```python
from build123d import *

# Parameters (mm, degrees)
SKETCH_1_W          = 10
SKETCH_1_H          = 10
EXTRUDE_1_DEPTH     = 2
EXTRUDE_2_DEPTH     = 3.3
SKETCH_3_R          = 2
CUT_EXTRUDE_1_DEPTH = 3.3
SKETCH_4_R          = 0.75
CUT_EXTRUDE_2_DEPTH = 3.3
SKETCH_5_R          = 1.5
CUT_EXTRUDE_3_DEPTH = 1
CUT_EXTRUDE_4_DEPTH = 9.836854644


with BuildPart() as part:
    # 草图1 → 凸台-拉伸1 (new body)
    with BuildSketch(Plane(origin=(0, 0, 0), x_dir=(1, 0, 0), z_dir=(0, 1, 0))):
        Rectangle(SKETCH_1_W, SKETCH_1_H)
    extrude(amount=EXTRUDE_1_DEPTH)

    # 草图2 → 凸台-拉伸2 (add)
    with BuildSketch(Plane.XZ):
        with BuildLine():
            ThreePointArc((-3.353126844, -0.498638517), (-2.397091988, -2.397091988), (-0.498638517, -3.353126844))
            ThreePointArc((-0.498638517, -3.353126844), (0, -2.89), (0.498638517, -3.353126844))
            ThreePointArc((0.498638517, -3.353126844), (2.397091988, -2.397091988), (3.353126844, -0.498638517))
            ThreePointArc((3.353126844, -0.498638517), (2.89, 0), (3.353126844, 0.498638517))
            ThreePointArc((3.353126844, 0.498638517), (2.397091988, 2.397091988), (0.498638517, 3.353126844))
            ThreePointArc((0.498638517, 3.353126844), (0, 2.89), (-0.498638517, 3.353126844))
            ThreePointArc((-0.498638517, 3.353126844), (-2.397091988, 2.397091988), (-3.353126844, 0.498638517))
            ThreePointArc((-3.353126844, 0.498638517), (-2.89, 0), (-3.353126844, -0.498638517))
        make_face()
    extrude(amount=EXTRUDE_2_DEPTH)

    # 草图3 → 切除-拉伸1 (cut)
    with BuildSketch(Plane.XZ.offset(3.3)):
        with Locations(Location((0, 0, 0), (0, 0, 270))):
            Circle(SKETCH_3_R)
    extrude(amount=-CUT_EXTRUDE_1_DEPTH, mode=Mode.SUBTRACT)

    # 草图4 → 切除-拉伸2 (cut)
    with BuildSketch(Plane.XZ):
        with Locations(Location((0, 0, 0), (0, 0, 270))):
            Circle(SKETCH_4_R)
    extrude(amount=-CUT_EXTRUDE_2_DEPTH, mode=Mode.SUBTRACT)

    # 草图5 → 切除-拉伸3 (cut)
    with BuildSketch(Plane(origin=(0, 2, 0), x_dir=(1, 0, 0), z_dir=(0, 1, 0))):
        with Locations(Location((0, 0, 0), (0, 0, 270))):
            Circle(SKETCH_5_R)
    extrude(amount=-CUT_EXTRUDE_3_DEPTH, mode=Mode.SUBTRACT)

    # 草图6 → 切除-拉伸4 (cut, through all)
    with BuildSketch(Plane(origin=(0, 2, 0), x_dir=(1, 0, 0), z_dir=(0, 1, 0))):
        with BuildLine():
            Line((-0.5, 5), (0.5, 5))
            ThreePointArc((0.5, 5), (0, 4.5), (-0.5, 5))
        make_face()
    extrude(amount=-CUT_EXTRUDE_4_DEPTH, mode=Mode.SUBTRACT)


solid = part.part
```
The listing builds one solid part. Answer for the finished solid, in the listing's coordinates (mm). A direction names the side the tool comes from. Coordinates: 2 decimals unless noted, no trailing zeros. Loops run counter-clockwise (first coordinate to the right, second up) from the corner with the lowest first, then second, coordinate; pieces in that order, holes last. Notation, with made-up numbers: (-25.75, -24.75) -> (19.25, -24.75) arc R26 cw to (19.25, -1.75) -> close; hole circle Ø3 at (66, -34.75). An arc over 180 degrees is marked (long way). Use one line per item in the form item = value. Start each with the question number.
Item 1: A tool of negligible diameter and unlimited length cuts with its end or side. For faces 1 (the face through (-2.376, -1.627, 2.418)), 2 (the face through (-2, -2, 0)), 3 (the face through (0.01, -1.63, 2.89)), from which of +Z, -Z, +X, -X, +Y, -Y can it reach the whole face along a straight path? Write none if from no direction.
Item 2: The part is cut by section D-D on y = -2. Determine the outline of the cut face in (x, z).
Item 3: Consider L1, parallel to Y at x = 3.5, z = -2.5; L2, parallel to Z at x = -0.25, y = -1.75; L3, parallel to Z at x = -0.75, y = -0.25. Determine where each line is inside the solid, lowest interval first. Write a range as [from, to].
Item 4: Flat-ended cylindrical pins translate along their axes: pin 1 Ø1.5 at (x, y) = (1.5, -2.5) entering from +Z; pin 2 Ø1.5 at (x, z) = (0.5, -0.5) entering from +Y; pin 3 Ø1.4 at (x, z) = (0, 0) entering from +Y. Find the tip coordinate at first contact, or state that the pin passes through.
Item 5: The part is cut by section C-C on x = 0. Determine the outline of the cut face in (y, z), then the cut area to 3 significant figures.
Item 6: The mould has two halves that part along X. Classify faces 4 (the face through (2.376, -1.627, -2.418)), 5 (the face through (-5, 1, 0)), 6 (the face through (0.225, 0.493, -0.715)): released by +X, released by -X, zero draft, split by the parting line, or undercut.
Item 7: The part is cut by section A-A on y = 1.3. Determine the outline of the cut face in (x, z).
Item 8: The part is cut by section B-B on z = 0. Determine the outline of the cut face in (x, y).
Answer key:
q1.face_1 = +Z, -X, -Y
q1.face_2 = -Y
q1.face_3 = +Z, -Y
q2.outline = (-3.35, -0.5) arc R3.39 ccw to (-0.5, -3.35) arc R0.5 cw to (0.5, -3.35) arc R3.39 ccw to (3.35, -0.5) arc R0.5 cw to (3.35, 0.5) arc R3.39 ccw to (0.5, 3.35) arc R0.5 cw to (-0.5, 3.35) arc R3.39 ccw to (-3.35, 0.5) arc R0.5 cw to start; hole circle Ø4 at (0, 0)
q3.L1 = [0, 2]
q3.L2 = [-2.96, -1.98], [1.98, 2.96]
q3.L3 = [-3.31, -1.85], [1.85, 3.31]
q4.pin_1 = 3.31
q4.pin_2 = 1
q4.pin_3 = through
q5.outline = (-3.3, -2.89) -> (0, -2.89) -> (0, -4.5) -> (2, -4.5) -> (2, -1.5) -> (1, -1.5) -> (1, -0.75) -> (0, -0.75) -> (0, -2) -> (-3.3, -2) -> close; (-3.3, 2) -> (0, 2) -> (0, 0.75) -> (1, 0.75) -> (1, 1.5) -> (2, 1.5) -> (2, 5) -> (0, 5) -> (0, 2.89) -> (-3.3, 2.89) -> close
q5.area = 20.4 mm2
q6.face_4 = released by +X
q6.face_5 = released by -X
q6.face_6 = undercut
q7.outline = (-5, -5) -> (-0.5, -5) arc R0.5 cw to (0.5, -5) -> (5, -5) -> (5, 5) -> (-5, 5) -> close; hole circle Ø3 at (0, 0)
q8.outline = (-5, 0) -> (-2.89, 0) -> (-2.89, -3.3) -> (-2, -3.3) -> (-2, 0) -> (-0.75, 0) -> (-0.75, 1) -> (-1.5, 1) -> (-1.5, 2) -> (-5, 2) -> close; (0.75, 0) -> (2, 0) -> (2, -3.3) -> (2.89, -3.3) -> (2.89, 0) -> (5, 0) -> (5, 2) -> (1.5, 2) -> (1.5, 1) -> (0.75, 1) -> close
